Autodesk Inventor part; units mm, degrees
ref_plane "YZ Plane" through (0, 0, 0) normal (1, 0, 0) x (0, 1, 0)
ref_plane "XZ Plane" through (0, 0, 0) normal (0, 1, 0) x (-1, 0, 0)
ref_plane "XY Plane" through (0, 0, 0) normal (0, 0, 1) x (1, 0, 0)
sketch "Sketch1" plane through (0, 0, 0) normal (0, 1, 0) x (-1, 0, 0)
  line L0 (4.0152, 32.5375) -> (-70.4848, 32.5375)
  line L1 (-70.4848, 32.5375) -> (-70.4848, -7.4625)
  line L2 (-70.4848, -7.4625) -> (4.0152, -7.4625)
  line L3 (4.0152, -7.4625) -> (4.0152, 32.5375)
  point P0 (0, 0)
  dimension "d0" = 74.5
  dimension "d1" = 40
extrude "Extrusion1" add sketch "Sketch1" along normal blind 75
sketch "Sketch3" plane through (0, 75, 0) normal (0, 1, 0) x (1, 0, 0)
  line L0 (-2.5152, 5.9625) -> (32.4848, 5.9625)
  line L1 (32.4848, 5.9625) -> (32.4848, -31.0375)
  line L2 (32.4848, -31.0375) -> (-2.5152, -31.0375)
  line L3 (-2.5152, -31.0375) -> (-2.5152, 5.9625)
  line L4 (33.9848, 5.9625) -> (68.9848, 5.9625)
  line L5 (68.9848, 5.9625) -> (68.9848, -31.0375)
  line L6 (68.9848, -31.0375) -> (33.9848, -31.0375)
  line L7 (33.9848, -31.0375) -> (33.9848, 5.9625)
  line L8 (70.4848, 7.4625) -> (-4.0152, 7.4625)
  line L9 (70.4848, -32.5375) -> (70.4848, 7.4625)
  line L10 (-4.0152, -32.5375) -> (70.4848, -32.5375)
  line L11 (-4.0152, 7.4625) -> (-4.0152, -32.5375)
  point P0 (0, 0)
  dimension "d10" = 1.5
  dimension "d11" = 1.5
  dimension "d12" = 1.5
  dimension "d13" = 1.5
  dimension "d14" = 1.5
  dimension "d15" = 35
  dimension "d16" = 35
extrude "Extrusion3" cut sketch "Sketch3" against normal blind 73.5 contours L4 L5 L6 L7
extrude "Extrusion4" cut sketch "Sketch3" against normal blind 73.5 contours L0 L1 L2 L3
equation "\"d11\" = d10"
equation "\"d12\" = d10"
equation "\"d14\" = d10"
equation "\"d15\" = d16"
properties part number "_3DPrint"
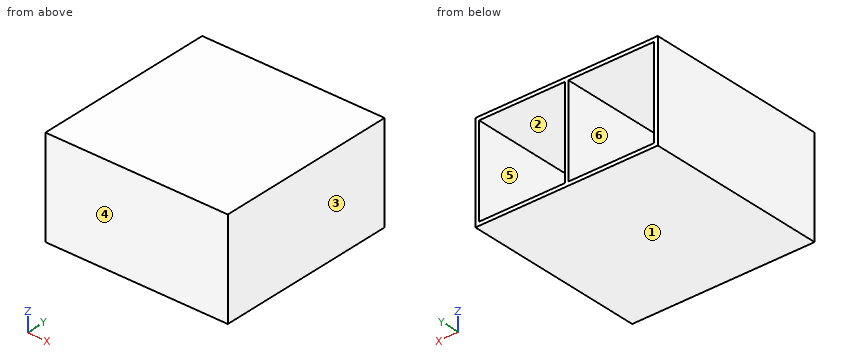
Verification items for the finished model (mm, model axes). Face numbers are marked on the shaded views. A direction names the side the tool comes from. Round coordinates to 2 decimals unless told otherwise and drop trailing zeros. Write each loop counter-clockwise with the first axis right and the second up, starting at its lowest first coordinate (ties: lowest second). Pieces come first, ordered by that corner, then holes. Notation, with made-up numbers: (-22, 42) - (20, 42) arc R21 cw to (20, 62) - close; hole circle Ø11 at (46.5, 11). An arc over 180 degrees is marked (long way). Answer as a JSON object with one key per item and string values. Group by question number.
Q1. Mould release check, pull along X, two halves, no side actions. Record for the marked faces 3, 4, 5 and 6: released by +X, released by -X, zero draft, split by the parting line, or undercut.
Q2. Thickness scan on line 1 (X direction, y = 31.5, z = 8.5); line 2 (Z direction, x = 17, y = 46); line 3 (Y direction, x = 27, z = 15.5). Record the ranges inside material, lowest first.
Q3. Section check C-C, the plane x = 31.5. Enter the section's corners in (y, z).
Q4. Tool access check on the marked faces 1 and 2. Record the directions out of +Z, -Z, +X, -X, +Y, -Y that give a thin tool (end or side, any length) a straight path to the whole face; none if there is none.
Q5. Section check A-A, the plane y = 8.5. Enter the section's corners in (x, z), plus the area to 3 significant figures.
Q6. Section check B-B, the plane z = 21. Enter the section's corners in (x, y).
Found:
{
 "1": {"face 3": "released by +X", "face 4": "zero draft", "face 5": "undercut", "face 6": "undercut"},
 "2": {"line 1": "x = -4.02 to -2.52, 32.48 to 33.98, 68.98 to 70.48", "line 2": "z = -7.46 to -5.96, 31.04 to 32.54", "line 3": "y = 0 to 1.5"},
 "3": {"outline": "(0, -7.46) - (75, -7.46) - (75, -5.96) - (1.5, -5.96) - (1.5, 31.04) - (75, 31.04) - (75, 32.54) - (0, 32.54) - close"},
 "4": {"face 1": "-Z, +X, -X, +Y, -Y", "face 2": "+Y"},
 "5": {"outline": "(-4.02, -7.46) - (70.48, -7.46) - (70.48, 32.54) - (-4.02, 32.54) - close; hole (-2.52, -5.96) - (32.48, -5.96) - (32.48, 31.04) - (-2.52, 31.04) - close; hole (33.98, -5.96) - (68.98, -5.96) - (68.98, 31.04) - (33.98, 31.04) - close", "area": "390 mm^2"},
 "6": {"outline": "(-4.02, 0) - (70.48, 0) - (70.48, 75) - (68.98, 75) - (68.98, 1.5) - (33.98, 1.5) - (33.98, 75) - (32.48, 75) - (32.48, 1.5) - (-2.52, 1.5) - (-2.52, 75) - (-4.02, 75) - close"}
}
